The model under review builds one solid part; all positions refer to its coordinate system, in mm. Give positions to 0.01 mm unless a question says otherwise; leave off trailing zeros. Write each loop counter-clockwise with the first axis right and the second up, starting at its lowest first coordinate (ties: lowest second). Pieces come first, ordered by that corner, then holes. Notation, with made-up numbers: (-31, -35.75) - (23, -35.75) arc R25 cw to (23, -7.75) - close; hole circle Ø1 at (88.5, 43). An arc over 180 degrees is marked (long way). Write item = value, one per line.
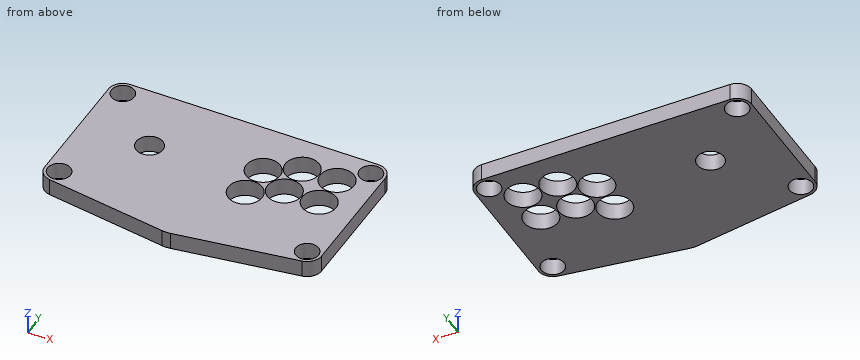
```python
from build123d import *

# Parameters (mm, degrees)
F0_R     = 12
F0_R_2   = 17.75
F0_R_3   = 14
F1_DEPTH = 18


with BuildPart() as f1:
    # F0 (on Top) → F1 (new body)
    with BuildSketch(Plane.XY):
        with BuildLine():
            ThreePointArc((145, 63.942884), (140.606602, 74.549485), (130, 78.942884))
            Line((130, 78.942884), (-130, 78.942884))
            ThreePointArc((-130, 78.942884), (-140.606602, 74.549485), (-145, 63.942884))
            Line((-145, 63.942884), (-145, -66.057116))
            ThreePointArc((-145, -66.057116), (-141.378114, -75.831498), (-132.261529, -80.885653))
            Line((-132.261529, -80.885653), (-4.523058, -100.367296))
            ThreePointArc((-4.523058, -100.367296), (0, -100.710224), (4.523058, -100.367296))
            Line((4.523058, -100.367296), (132.261529, -80.885653))
            ThreePointArc((132.261529, -80.885653), (141.378114, -75.831498), (145, -66.057116))
            Line((145, -66.057116), (145, 63.942884))
        make_face()
        with Locations((-130, -66.057116)):
            Circle(F0_R, mode=Mode.SUBTRACT)
        with Locations((130, -66.057116)):
            Circle(F0_R, mode=Mode.SUBTRACT)
        with Locations((38.445036, -14.252153)):
            Circle(F0_R_2, mode=Mode.SUBTRACT)
        with Locations((-72.5, 6.442884)):
            Circle(F0_R_3, mode=Mode.SUBTRACT)
        with Locations((-130, 63.942884)):
            Circle(F0_R, mode=Mode.SUBTRACT)
        with Locations((70.054964, 3.997847)):
            Circle(F0_R_2, mode=Mode.SUBTRACT)
        with Locations((38.445036, 22.247847)):
            Circle(F0_R_2, mode=Mode.SUBTRACT)
        with Locations((106.554964, 3.997847)):
            Circle(F0_R_2, mode=Mode.SUBTRACT)
        with Locations((70.054964, 40.497847)):
            Circle(F0_R_2, mode=Mode.SUBTRACT)
        with Locations((106.554964, 40.497847)):
            Circle(F0_R_2, mode=Mode.SUBTRACT)
        with Locations((130, 63.942884)):
            Circle(F0_R, mode=Mode.SUBTRACT)
    extrude(amount=F1_DEPTH)


solid = f1.part
```
1. Insertion check: P1, Ø6, axis at x = 99, z = 5.5, coming from the -Y side; P2, Ø14.5, axis at x = -130, y = -66.06, coming from the -Z side; P3, Ø8, axis at x = 14.5, z = 5.5, coming from the -Y side. Each pin has a flat end and moves straight along its axis. Give the tip position at first contact, or say it passes through.
Findings below:
P1 = -86.42
P2 = through
P3 = -99.46
2. Take a section at B-B on y = 68. Give the boundary of the cut face in (x, z), and give its area (3 significant figures).
Findings below:
outline = (-144.44, 0) - (-141.29, 0) - (-141.29, 18) - (-144.44, 18) - close; (-118.71, 0) - (118.71, 0) - (118.71, 18) - (-118.71, 18) - close; (141.29, 0) - (144.44, 0) - (144.44, 18) - (141.29, 18) - close
area = 4,390 mm²
3. For line 1 (Y direction, x = 84, z = 15); line 2 (Y direction, x = 110, z = 9); line 3 (X direction, y = 18, z = 4.75), list the stretches that pass through material, from the lowest coordinate up. Write a range as from..to.
Findings below:
line_1 = -88.25..-6.98, 14.98..29.52, 51.48..78.94
line_2 = -84.28..-13.41, 21.41..23.09, 57.91..78.94
line_3 = -145..-80.4, -64.6..21.21, 55.68..59.15, 80.96..95.65, 117.46..145
4. Take a section at A-A on x = -72.5. Give the boundary of the cut face in (y, z).
Findings below:
outline = (-90, 0) - (-7.56, 0) - (-7.56, 18) - (-90, 18) - close; (20.44, 0) - (78.94, 0) - (78.94, 18) - (20.44, 18) - close
5. Take a section at D-D on x = -106.5. Give the boundary of the cut face in (y, z), and give its area (3 significant figures).
Findings below:
outline = (-84.81, 0) - (78.94, 0) - (78.94, 18) - (-84.81, 18) - close
area = 2,950 mm²
6. Take a section at C-C on z = 6.75. Count the separate pieces of the cut face and the enclosed holes in it, and give its area (3 significant figures).
Findings below:
separate_pieces = 1
enclosed_holes = 11
area = 40,500 mm²
